from build123d import *

# Parameters (mm, degrees)
SKETCH_1_R             = 5.1
SKETCH_1_R_2           = 3.1
SM_BASE_FLANGE_1_DEPTH = 4
SKETCH_29_R            = 2.1
CUT_EXTRUDE_7_DEPTH    = 10
CUT_EXTRUDE_11_DEPTH   = 10


# Sheet-metal steps are written as plain solids
with BuildPart() as part:
    # Sketch 1 → Базовая кромка1 (new body)
    with BuildSketch(Plane.XY):
        with BuildLine():
            Line((21.416256147, 65.130237954), (-13.484101554, 6.571073374))
            ThreePointArc((-13.484101554, 6.571073374), (-12.719396617, -7.950908734), (0, -15))
            ThreePointArc((0, -15), (110.130832642, -5.633175847), (220.379871586, -13.487289734))
            ThreePointArc((220.379871586, -13.487289734), (223.626784147, -14.026708962), (226.855383886, -14.666676157))
            ThreePointArc((226.855383886, -14.666676157), (228.418883679, -14.916436276), (230, -15))
            ThreePointArc((230, -15), (244.896230479, -1.761339697), (233.49830961, 14.586357663))
            Line((233.49830961, 14.586357663), (31.656582874, 69.861832141))
            ThreePointArc((31.656582874, 69.861832141), (25.805552993, 69.077808893), (21.416256147, 65.130237954))
        make_face()
        Circle(SKETCH_1_R, mode=Mode.SUBTRACT)
        with Locations((230, 0)):
            Circle(SKETCH_1_R, mode=Mode.SUBTRACT)
        with Locations((30, 60)):
            Circle(SKETCH_1_R_2, mode=Mode.SUBTRACT)
        with BuildLine():
            Line((37.603385022, 47.496856423), (130.332311604, 22.102526432))
            ThreePointArc((130.332311604, 22.102526432), (133.234743351, 17.673003854), (129.197928501, 14.245336107))
            ThreePointArc((129.197928501, 14.245336107), (73.556484101, 13.205174657), (18.156304087, 7.92574997))
            ThreePointArc((18.156304087, 7.92574997), (14.286499385, 9.687372505), (14.189161482, 13.938163928))
            Line((14.189161482, 13.938163928), (33.110820822, 45.686737192))
            ThreePointArc((33.110820822, 45.686737192), (35.05198474, 47.349074558), (37.603385022, 47.496856423))
        make_face(mode=Mode.SUBTRACT)
    extrude(amount=-SM_BASE_FLANGE_1_DEPTH)

    # Эскиз29 → Вырез-Вытянуть7 (cut)
    with BuildSketch(Plane.XY):
        with Locations((116.790365799, 36.179268785)):
            Circle(SKETCH_29_R)
        with Locations((174.659589105, 20.331461556)):
            Circle(SKETCH_29_R)
        with Locations((58.921142493, 52.027076013)):
            Circle(SKETCH_29_R)
        with Locations((57.341971973, 2.442823407)):
            Circle(SKETCH_29_R)
        with Locations((145.69468633, 4.101167629)):
            Circle(SKETCH_29_R)
    extrude(amount=-CUT_EXTRUDE_7_DEPTH, mode=Mode.SUBTRACT)

    # Эскиз47 → Вырез-Вытянуть11 (cut)
    with BuildSketch(Plane.XY):
        with BuildLine():
            ThreePointArc((186.876285814, 1.505913283), (189.914433505, -1.752101237), (193.172448024, 1.286046453))
            ThreePointArc((193.172448024, 1.286046453), (193.709834302, 6.398935347), (194.953567375, 11.387276243))
            ThreePointArc((194.953567375, 11.387276243), (192.93114288, 15.356507801), (188.961911322, 13.334083307))
            ThreePointArc((188.961911322, 13.334083307), (187.505545458, 7.492918866), (186.876285814, 1.505913283))
        make_face()
    extrude(amount=-CUT_EXTRUDE_11_DEPTH, mode=Mode.SUBTRACT)


solid = part.part
Geometry: final body of the model. Coordinates: model frame, mm. A direction names the side the tool comes from. Round coordinates to 2 decimals unless told otherwise and drop trailing zeros. Loops run counter-clockwise (first coordinate to the right, second up) from the corner with the lowest first, then second, coordinate; pieces in that order, holes last.
Q1. Pull-direction query (Y, two-part tool) for faces 1 (the flat face through (113, 28, 0)), 2 (the cylindrical face through (14.32, 9.64, -1.97)), 3 (the cylindrical face through (108.582, -5.645, -1.972)); classes: released by +Y, released by -Y, zero draft, split by the parting line, or undercut.
Q2. Section D-D on x = 158. Return loops of the section in (y, z).
Q3. Pin query (flat end, axial travel): P1, Ø2.5, axis at x = 58.92, y = 52.03, coming from the +Z side. Return the tip coordinate at first contact, or that it passes through.
Q4. Material intervals for L1, parallel to X at y = -1, z = -2.5; L2, parallel to X at y = -0.5, z = -1.75; L3, parallel to Y at x = 230, z = -1.6, sorted ascending.
Q5. Access query for faces 4 (the flat face through (83.319, 34.977, -1.972)), 5 (the flat face through (133.99, 41.837, -1.972)). Directions: +Z, -Z, +X, -X, +Y, -Y. A direction counts if a zero-diameter tool reaches every point of the face in a straight line with its end or side. Return the directions, or none.
Q6. Section A-A on y = 60. Return loops of the section in (x, z), plus the area to 3 significant figures.
Q7. Section C-C on x = 96. Return loops of the section in (y, z).
Q8. Section B-B on z = -3. State how many separate pieces and enclosed holes the cut face has, plus the area to 3 significant figures.
Evaluation:
1. face 1: zero draft
1. face 2: undercut
1. face 3: released by -Y
2. outline: (-6.92, -4) - (35.26, -4) - (35.26, 0) - (-6.92, 0) - close
3. P1: passes through
4. L1: x = -14.97 to -5, 5 to 187.98, 192.07 to 225, 235 to 244.97
4. L2: x = -14.99 to -5.08, 5.08 to 187.51, 192.54 to 224.92, 235.08 to 244.99
4. L3: y = -15 to -5.1, 5.1 to 15.54
5. face 4: +Z, -Z
5. face 5: +Z, -Z, +X, +Y
6. outline: (18.36, -4) - (26.9, -4) - (26.9, 0) - (18.36, 0) - close; (33.1, -4) - (67.67, -4) - (67.67, 0) - (33.1, 0) - close
6. area: 172 mm2
7. outline: (-5.87, -4) - (14.14, -4) - (14.14, 0) - (-5.87, 0) - close; (31.5, -4) - (52.24, -4) - (52.24, 0) - (31.5, 0) - close
8. separate pieces: 1
8. enclosed holes: 10
8. area: 10,000 mm2
